Autodesk Inventor part; units mm, degrees
ref_plane "Work Plane1" through (104.775, 0, 0) normal (0, 0, -1) x (1, 0, 0)
ref_plane "YZ Plane" through (0, 0, 0) normal (1, 0, 0) x (0, 1, 0)
ref_plane "XZ Plane" through (0, 0, 0) normal (0, 1, 0) x (-1, 0, 0)
sketch "Skizze1" plane through (0, 0, 0) normal (0, 0, 1) x (1, 0, 0)
  line L0 (4, 0) -> (4, 1.5)
  line L1 (4, 1.5) -> (3, 1.5)
  line L2 (3, 1.5) -> (2.6933, 1.5)
  line L3 (0, 2.77) -> (0, 1.1547)
  line L4 (0, 1.1547) -> (1.3, 1.1547)
  line L5 (1.3, 1.1547) -> (1.9667, 0)
  line L6 (1.9667, 0) -> (4, 0)
  line L7 (0, 2.77) -> (0.59, 2.77)
  line L8 (0.59, 2.77) -> (1.86, 1.5)
  line L9 (2.6933, 1.5) -> (1.86, 1.5)
  line L10 (3, 1.5) -> (1.86, 1.5) construction
  line L11 (1.86, 1.5) -> (1.86, 1.5)
  line L12 (-0.8, 0) -> (4.8, 0)
  line L13 (0, -0.554) -> (0, 3.324)
  dimension "d0" = 4
  dimension "d1" = 1
  dimension "d2" = 1.3
  dimension "d3" = 3
  dimension "d6" = 1.86
  dimension "d7" = 45
  dimension "d8" = 2.3094
  dimension "d9" = 60
  dimension "d10" = 5.54
  dimension "d11" = 3
  dimension "d12" = 0.3067
revolve "Körper" add sketch "Skizze1" angle 360 about axis through (1.9667, 0, 0) along (1, 0, 0) contours L6 L5 L4 L3 L7 L8 L9 L2 L1 L0
sketch "Skizze2" plane through (0, 0, 0) normal (-1, 0, 0) x (0, 0, 1)
  circle A0 centre (0, 0) radius 1.1547
  line L0 (0, -3.878) -> (0, 3.878)
  line L1 (-3.878, 0) -> (3.878, 0)
  line L2 (1.1547, 0) -> (0.5774, -1)
  line L3 (0.5774, -1) -> (-0.5774, -1)
  line L4 (-0.5774, -1) -> (-1.1547, 0)
  line L5 (-1.1547, 0) -> (-0.5774, 1)
  line L6 (-0.5774, 1) -> (0.5774, 1)
  line L7 (0.5774, 1) -> (1.1547, 0)
  point P0 (0, 1.1547)
extrude "Loch" add sketch "Skizze2" against normal up to next contours L7 A0 | A0 L2 | L6 L0 A0 | A0 L0 L3 | L0 L6 A0 | A0 L3 L0 | L4 A0 | A0 L5
thread "Gewinde"
chamfer "Fase1" distance 0.3067 distance2 0.3067 1 edges at (4, -1.5, 0) measured on face at (4, 0.6824, 0.2556)
ref_plane "Work Plane1" through (104.775, 0, 0) normal (0, 0, -1) x (1, 0, 0)
equation "\"d15\" = GEL"
equation "\"d17\" = -0.5 * SPD + 0.5 * GD"
equation "\"d18\" = GUL"
equation "\"d2\" = INTI"
equation "\"d3\" = GD"
equation "\"d6\" = KOH"
equation "\"d7\" = 0.5 * SEWI"
equation "\"d8\" = 1.1547 * SW"
equation "\"d10\" = KOD"
equation "\"d11\" = BDM"
equation "\"d12\" = GAL"
equation "\"NLG\" = 8"
equation "\"INTI\" = 1.3"
equation "\"GEL\" = 4"
equation "\"GAL\" = 0.61345 * PTC"
equation "\"KOH\" = 1.86"
equation "\"KOD\" = 5.54"
equation "\"GUL\" = 0.61345 * PTC"
equation "\"SPD\" = NND - 1.2269 * PTC"
equation "\"BDM\" = NND"
equation "\"GD\" = NND"
equation "\"SEWI\" = 90deg"
equation "\"SW\" = 2"
equation "\"TOA\" = 30deg"
equation "\"GD1\" = THREADDIA - 1.2269 * PTC"
equation "\"EPV\" = 3.36"
equation "\"THREADDIA\" = 3"
equation "\"PTC\" = 0.5"
equation "\"NND\" = 3"
equation "\"E0\" = 2.31"
equation "\"THREADDESC\" = 1.2345"
properties part number "ISO 10642 - M3 x  8" material "Stahl"
Work out the finished part from the listing and answer in its coordinate system (mm). A direction names the side the tool comes from. Give positions to 0.01 mm unless a question says otherwise; leave off trailing zeros. Loops run counter-clockwise (first coordinate to the right, second up) from the corner with the lowest first, then second, coordinate; pieces in that order, holes last. Notation, with made-up numbers: (60, -32.5) - (118, -32.5) arc R14 cw to (118, -12.5) - close; hole circle Ø6 at (-36.75, -15). An arc over 180 degrees is marked (long way). One line per question, with ' | ' between items.
(1) Straight lines are drawn through the part: probe 1 along X at (y, z) = (-1, 1.7); probe 2 along Y at (x, z) = (1.25, -0.4); probe 3 along Z at (x, y) = (0.3, -1.65). For each, find the intervals that lie inside material, in ascending order.
Recorded:
probe 1: x = 0 to 1.39 | probe 2: y = -2.07 to -1, 1 to 2.07 | probe 3: z = -2.22 to 2.22
(2) The mould has two halves that part along Y. Classify faces 1 (the face through (1, -1, 0)), 2 (the face through (2.76, -1.5, -0.07)), 3 (the face through (0.68, 0.51, 0.86)), 4 (the face through (0, -1.2, 0)): +Y half, -Y half, draft (parallel to the pull), parting line (faces both ways), or undercut.
Recorded:
face 1: undercut | face 2: parting line | face 3: undercut | face 4: draft
(3) The part is cut by section A-A (x = 1.2). Write down the section's boundary in (y, z).
Recorded:
outline: circle Ø4.32 at (0, 0); hole (-1, -0.58) - (0, -1.15) - (1, -0.58) - (1, 0.58) - (0, 1.15) - (-1, 0.58) - close
(4) Each of these flat-tipped pins is pushed along its axis until it touches: pin 1 Ø3 at (y, z) = (0, -1.5) entering from -X; pin 2 Ø1 at (x, y) = (2.5, 0.5) entering from -Z. Where does it stop, or does it pass through?
Recorded:
pin 1: stops at x = 0 | pin 2: stops at z = -1.5
(5) A tool of negligible diameter and unlimited length cuts with its end or side. For faces 5 (the face through (4, 0, 0)), 6 (the face through (0.68, -0.51, -0.86)), from which of +Z, -Z, +X, -X, +Y, -Y can it reach the whole face along a straight path? Write none if from no direction.
Recorded:
face 5: +Z, -Z, +X, +Y, -Y | face 6: -X
